from build123d import *

# Parameters (mm, degrees)
ESBO_O1_W                      = 30
ESBO_O1_H                      = 14
FLANGE_BASE1_DEPTH             = 2
ARESTA_FLANGE1_STRIP_W         = 10
ARESTA_FLANGE1_STRIP_H         = 2
ARESTA_FLANGE1_STRIP_CUT_DEPTH = 30
ARESTA_FLANGE1_DEPTH           = 30
ESBO_O10_R                     = 1.25
CORTE_EXTRUS_O1_DEPTH          = 2
ESBO_O11_R                     = 1.25
CORTE_EXTRUS_O2_DEPTH          = 2
CHANFRO1_SIZE                  = 1.5
CORTE_EXTRUS_O3_DEPTH          = 2
FILETE1_R                      = 2


# Sheet-metal steps are written as plain solids
with BuildPart() as part:
    # Esboço1 → Flange-base1 (new body)
    with BuildSketch(Plane(origin=(0, 0, 0), x_dir=(0, 0, -1), z_dir=(1, 0, 0))):
        Rectangle(ESBO_O1_W, ESBO_O1_H)
    extrude(amount=-FLANGE_BASE1_DEPTH)

    # Aresta-Flange1 strip (across the edge) → Aresta-Flange1 strip cut (cut)
    with BuildSketch(Plane(origin=(0, -7, 15), x_dir=(0, 1, 0), z_dir=(0, 0, -1))):
        with Locations((-4, -1)):
            Rectangle(ARESTA_FLANGE1_STRIP_W, ARESTA_FLANGE1_STRIP_H)
    extrude(amount=ARESTA_FLANGE1_STRIP_CUT_DEPTH, mode=Mode.SUBTRACT)

    # Aresta-Flange1 section (across the edge) → Aresta-Flange1 (add)
    with BuildSketch(Plane(origin=(0, -7, 15), x_dir=(0, 1, 0), z_dir=(0, 0, -1))):
        with BuildLine():
            Line((-2, 1), (-2, 24))
            Line((-2, 24), (0, 24))
            Line((0, 24), (0, 1))
            ThreePointArc((0, 1), (0.292893219, 0.292893219), (1, 0))
            Line((1, 0), (1, -2))
            ThreePointArc((1, -2), (-1.121320344, -1.121320344), (-2, 1))
        make_face()
    extrude(amount=ARESTA_FLANGE1_DEPTH)

    # Esboço10 → Corte-extrusão1 (cut)
    with BuildSketch(Plane(origin=(0, 0, 0), x_dir=(0, 0, -1), z_dir=(1, 0, 0))):
        with Locations((-13, -1.3)):
            Circle(ESBO_O10_R)
        with Locations((9, -1.3)):
            Circle(ESBO_O10_R)
    extrude(amount=-CORTE_EXTRUS_O1_DEPTH, mode=Mode.SUBTRACT)

    # Esboço11 → Corte-extrusão2 (cut)
    with BuildSketch(Plane(origin=(0, -7, 0), x_dir=(1, 0, 0), z_dir=(0, 1, 0))):
        with Locations(Location((18, -10, 0), (0, 0, 180))):
            Circle(ESBO_O11_R)
        with Locations(Location((18, 12, 0), (0, 0, 180))):
            Circle(ESBO_O11_R)
    extrude(amount=-CORTE_EXTRUS_O2_DEPTH, mode=Mode.SUBTRACT)

    # Chanfro1
    chanfro1_edges = [part.edges().sort_by_distance(p)[0] for p in [
        (24, -8, 15),
    ]]
    chamfer(chanfro1_edges, length=CHANFRO1_SIZE)

    # Esboço12 → Corte-extrusão3 (cut)
    with BuildSketch(Plane(origin=(0, -7, 0), x_dir=(1, 0, 0), z_dir=(0, 1, 0))):
        with BuildLine():
            Line((19.828427125, -2.5), (24, -2.5))
            Line((24, -2.5), (24, 2.5))
            Line((24, 2.5), (20.414213562, -1.085786438))
            ThreePointArc((20.414213562, -1.085786438), (19.98066806, -1.734633135), (19.828427125, -2.5))
        make_face()
        with BuildLine():
            Line((24, -7.5), (24, -2.5))
            Line((24, -2.5), (19.828427125, -2.5))
            ThreePointArc((19.828427125, -2.5), (19.98066806, -3.265366865), (20.414213562, -3.914213562))
            Line((20.414213562, -3.914213562), (24, -7.5))
        make_face()
    extrude(amount=-CORTE_EXTRUS_O3_DEPTH, mode=Mode.SUBTRACT)

    # Filete1
    filete1_edges = [part.edges().sort_by_distance(p)[0] for p in [
        (24, -8, -2.5),
        (24, -8, 7.5),
    ]]
    fillet(filete1_edges, radius=FILETE1_R)


solid = part.part
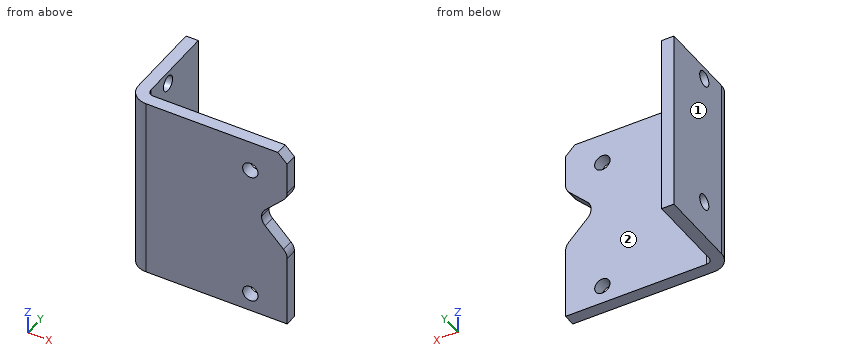
Could you check a few things on this model? Use its own coordinates, in mm. Face numbers are marked on the shaded views. A direction names the side the tool comes from. Give positions to 0.01 mm unless a question says otherwise; leave off trailing zeros. Order: outer loops, then holes, each group sorted by start corner. A loop starts at its lowest first (then second) coordinate and runs counter-clockwise, first axis right, second up. Notation, with made-up numbers: (39, 57) - (89, 57) arc R14 ccw to (89, 82) - close; hole circle Ø1 at (70, 75.5). An arc over 180 degrees is marked (long way). One line per question, with ' | ' between items. Start each with the question number.
Item 1: I'm going to push flat-ended pins straight in: pin 1 Ø1 at (y, z) = (2.5, -7) entering from +X; pin 2 Ø1 at (y, z) = (-1.5, -9) entering from -X; pin 3 Ø3 at (x, z) = (18, 10) entering from +Y. Where does each tip first touch, or does it pass through?
Item 2: I want a section at B-B on y = -1.3. Write out the boundary of the cut face in (x, z).
Item 3: I need wall thicknesses on probe 1 along Z at (x, y) = (18, -7.75); probe 2 along Y at (x, z) = (19.75, 5); probe 3 along X at (y, z) = (-4.75, 6.5). Which ranges of each line are inside material? Lowest first, please. Write a range as [from, to].
Item 4: I want a section at D-D on z = 4.5. Write out the boundary of the cut face in (x, y).
Item 5: I want a section at A-A on z = 10. Write out the boundary of the cut face in (x, y), then the cut area to 3 significant figures.
Item 6: For the marked faces 1 and 2, which set-ups out of +Z, -Z, +X, -X, +Y, -Y let a thin tool reach every point of the face, with its end or its side?
Item 7: I want a section at C-C on x = 18. Write out the boundary of the cut face in (y, z), then the cut area to 3 significant figures.
Verdict:
1) pin 1: x = 0 | pin 2: through | pin 3: y = -7
2) outline: (-2, -15) - (0, -15) - (0, -10.25) - (-2, -10.25) - close; (-2, -7.75) - (0, -7.75) - (0, 11.75) - (-2, 11.75) - close; (-2, 14.25) - (0, 14.25) - (0, 15) - (-2, 15) - close
3) probe 1: [-15, -13.25], [-10.75, 8.75], [11.25, 15] | probe 2: [-9, -7] | probe 3: [-2, 0]
4) outline: (-2, -6) arc R3 ccw to (1, -9) - (21, -9) - (21, -7) - (1, -7) arc R1 cw to (0, -6) - (0, 7) - (-2, 7) - close
5) outline: (-2, -6) arc R3 ccw to (1, -9) - (16.75, -9) - (16.75, -7) - (1, -7) arc R1 cw to (0, -6) - (0, 7) - (-2, 7) - close; (19.25, -9) - (24, -9) - (24, -7) - (19.25, -7) - close | area: 73.3 mm^2
6) face 1: +Z, -Z, -X, +Y, -Y | face 2: +Z, -Z, +X, +Y
7) outline: (-9, -15) - (-7, -15) - (-7, -13.25) - (-9, -13.25) - close; (-9, -10.75) - (-7, -10.75) - (-7, 8.75) - (-9, 8.75) - close; (-9, 11.25) - (-7, 11.25) - (-7, 15) - (-9, 15) - close | area: 50.0 mm^2
